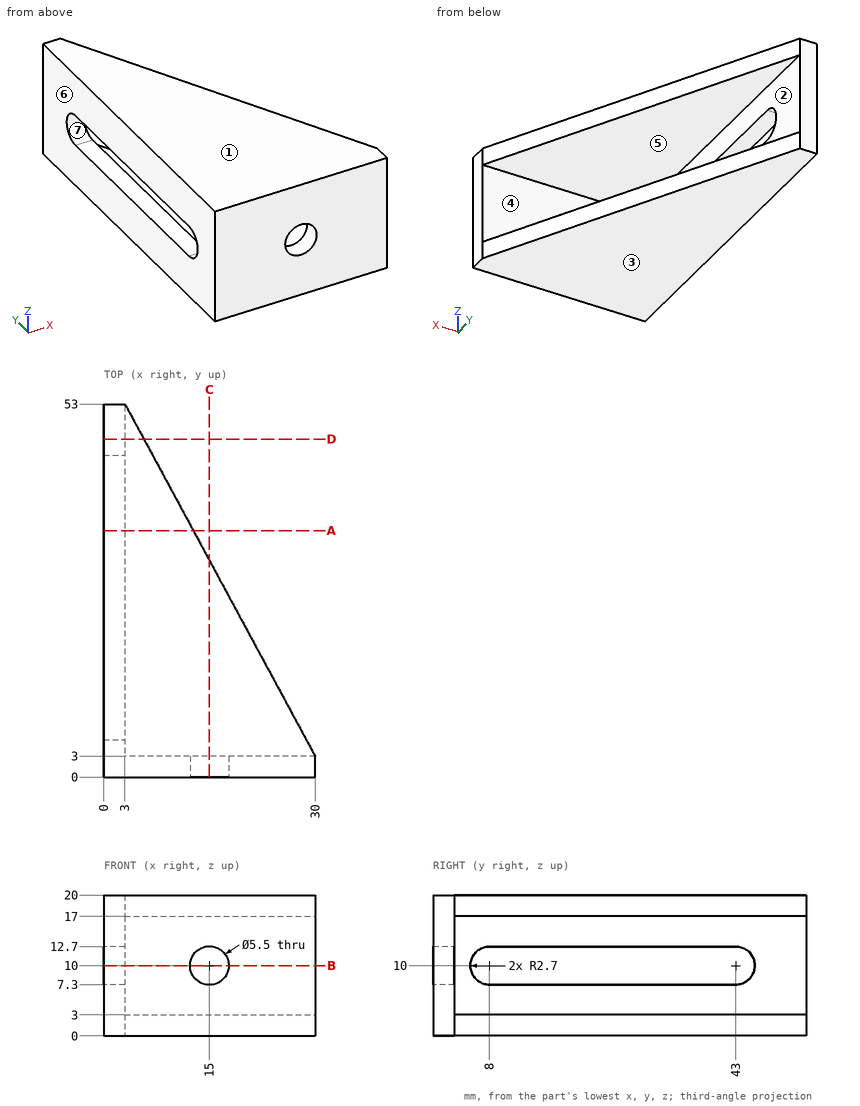
The figure shows three views and two pictorial views of one solid part (mm, origin at its lowest corner). Answer the questions. A direction names the side the tool comes from. Coordinates: 2 decimals unless noted, no trailing zeros. Write each loop counter-clockwise with the first axis right and the second up, starting at its lowest first coordinate (ties: lowest second). Pieces come first, ordered by that corner, then holes.
1. Consider line 1 along X through (y, z) = (2.35, 10); line 2 along Z through (x, y) = (2, 30); line 3 along Z through (x, y) = (14.5, 9). Determine where each line is inside the solid, lowest interval first.
Results list:
line 1: x = 0 to 12.25, 17.75 to 30
line 2: z = 0 to 7.3, 12.7 to 20
line 3: z = 0 to 3, 17 to 20
2. The part is cut by section D-D, the plane y = 48. Write down the section's boundary in (x, z), and give its area (3 significant figures).
Results list:
outline: (0, 0) - (5.7, 0) - (5.7, 3) - (3, 3) - (3, 17) - (5.7, 17) - (5.7, 20) - (0, 20) - close
area: 76.2 mm2
3. For the marked faces 5, 6 and 7, determine the directions among +Z, -Z, +X, -X, +Y, -Y from which every point of the face is accessible in a straight line to the end or side of a thin tool.
Results list:
face 5: +X, +Y
face 6: +Z, -Z, -X, +Y, -Y
face 7: +X, -X
4. For a pull along Z with two mould halves and no side action, classify the marked faces 1, 2, 3 and 4 as +Z half, -Z half, draft (parallel to the pull), parting line (faces both ways), or undercut.
Results list:
face 1: +Z half
face 2: undercut
face 3: -Z half
face 4: undercut
5. The part is cut by section B-B, the plane z = 10. Write down the section's boundary in (x, y).
Results list:
outline: (0, 0) - (12.25, 0) - (12.25, 3) - (3, 3) - (3, 5.3) - (0, 5.3) - close; (0, 45.7) - (3, 45.7) - (3, 53) - (0, 53) - close; (17.75, 0) - (30, 0) - (30, 3) - (17.75, 3) - close
6. Flat-ended cylindrical pins translate along their axes: pin 1 (1.5 mm diameter, centred on x = 14, z = 15, fed in from +Y); pin 2 (1.5 mm diameter, centred on y = 41, z = 6.5, fed in from +X). Find the tip coordinate at first contact, or state that the pin passes through.
Results list:
pin 1: stops at y = 3
pin 2: stops at x = 3
7. The part is cut by section C-C, the plane x = 15. Write down the section's boundary in (y, z), and give its area (3 significant figures).
Results list:
outline: (0, 0) - (30.78, 0) - (30.78, 3) - (3, 3) - (3, 7.25) - (0, 7.25) - close; (0, 12.75) - (3, 12.75) - (3, 17) - (30.78, 17) - (30.78, 20) - (0, 20) - close
area: 210 mm2
8. The part is cut by section A-A, the plane y = 35. Write down the section's boundary in (x, z).
Results list:
outline: (0, 0) - (12.72, 0) - (12.72, 3) - (3, 3) - (3, 7.3) - (0, 7.3) - close; (0, 12.7) - (3, 12.7) - (3, 17) - (12.72, 17) - (12.72, 20) - (0, 20) - close
